from build123d import *

# Parameters (mm, degrees)
SKETCH1_W           = 250
SKETCH1_H           = 250
BOSS_EXTRUDE1_DEPTH = 20
SKETCH2_W           = 40
SKETCH2_H           = 40
SKETCH2_W_2         = 30
SKETCH2_H_2         = 15
CUT_EXTRUDE2_DEPTH  = 5


with BuildPart() as part:
    # Sketch1 → Boss-Extrude1 (new body)
    with BuildSketch(Plane.XY):
        with Locations((22.048407602, -70.903707865)):
            Rectangle(SKETCH1_W, SKETCH1_H)
    extrude(amount=BOSS_EXTRUDE1_DEPTH)

    # Sketch2 → Cut-Extrude2 (cut)
    with BuildSketch(Plane.XY.offset(20)):
        Polygon((95.548407602, -105.403707865), (110.548407602, -105.403707865), (110.548407602, -90.403707865), (110.548407602, -75.403707865), (95.548407602, -75.403707865), align=None)
        with Locations((22.048407602, -70.903707865)):
            Rectangle(SKETCH2_W, SKETCH2_H)
        with Locations((41.548407602, 10.096292135)):
            Rectangle(SKETCH2_W_2, SKETCH2_H_2)
    extrude(amount=-CUT_EXTRUDE2_DEPTH, mode=Mode.SUBTRACT)


solid = part.part
The model under review builds one solid part; all positions refer to its coordinate system, in mm. A direction names the side the tool comes from. Coordinates: 2 decimals unless noted, no trailing zeros. Order: outer loops, then holes, each group sorted by start corner. A loop starts at its lowest first (then second) coordinate and runs counter-clockwise, first axis right, second up. Notation, with made-up numbers: (40, 34) -> (62, 34) arc R18 cw to (62, 47) -> close; hole circle Ø11 at (34.5, 52). An arc over 180 degrees is marked (long way). Answer in a Markdown table with one row per item.
(1) Consider section B-B (y = -100.5). Write out the cut boundary in (x, z), plus the area to 4 significant figures.
Answers:
| item | result |
|---|---|
| outline | (-102.95, 0) -> (147.05, 0) -> (147.05, 20) -> (110.55, 20) -> (110.55, 15) -> (95.55, 15) -> (95.55, 20) -> (-102.95, 20) -> close |
| area | 4,925 mm² |
(2) Consider section A-A (x = 30). Write out the cut boundary in (y, z), plus the area to 4 significant figures.
Answers:
| item | result |
|---|---|
| outline | (-195.9, 0) -> (54.1, 0) -> (54.1, 20) -> (17.6, 20) -> (17.6, 15) -> (2.6, 15) -> (2.6, 20) -> (-50.9, 20) -> (-50.9, 15) -> (-90.9, 15) -> (-90.9, 20) -> (-195.9, 20) -> close |
| area | 4,725 mm² |
(3) Machinability: for faces 1 (the flat face through (41, 10, 15)), 2 (the flat face through (147.048, -73, 10)), which of the approach directions +Z, -Z, +X, -X, +Y, -Y give a long, thin tool a straight path to every point of the face, cutting with its end or side? Answer none if there is none.
Answers:
| item | result |
|---|---|
| face 1 | +Z |
| face 2 | +Z, -Z, +X, +Y, -Y |
(4) The part is to be moulded in two halves that separate along Y. For faces 3 (the flat face through (-7, -69, 20)), 4 (the flat face through (103, -90, 15)), 5 (the flat face through (20, 54.096, 10)), say which applies: +Y half, -Y half, draft (parallel to the pull), parting line (faces both ways), or undercut.
Answers:
| item | result |
|---|---|
| face 3 | draft |
| face 4 | undercut |
| face 5 | +Y half |
